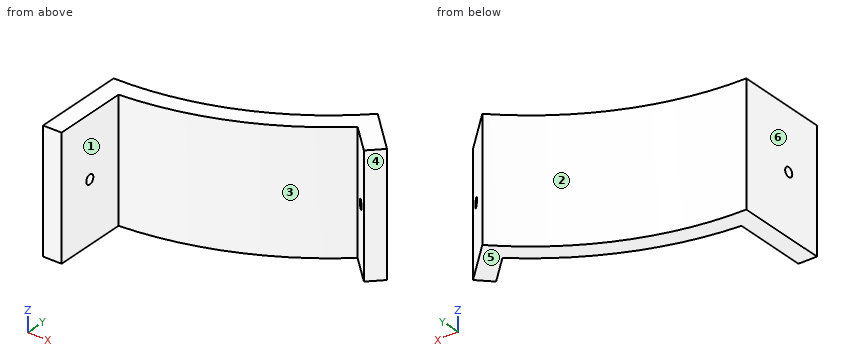
from build123d import *

# Parameters (mm, degrees)
SALIENTE_EXTRUIR1_DEPTH = 65.25
CROQUIS5_R              = 2.5
CORTAR_EXTRUIR3_DEPTH   = 45
CROQUIS6_R              = 2.5
CORTAR_EXTRUIR4_DEPTH   = 12


with BuildPart() as part:
    # Croquis1 → Saliente-Extruir1 (new body)
    with BuildSketch(Plane.XY):
        with BuildLine():
            Line((129.342755363, -129.342755363), (108.187337522, -108.187337522))
            ThreePointArc((108.187337522, -108.187337522), (58.550565152, -141.353568474), (0, -153))
            Line((0, -153), (0, -163))
            Line((0, -163), (0, -203))
            Line((0, -203), (10, -203))
            Line((10, -203), (10, -162.692962355))
            ThreePointArc((10, -162.692962355), (62.377399476, -150.592363799), (107.970229121, -122.112364745))
            Line((107.970229121, -122.112364745), (122.271687551, -136.413823175))
            Line((122.271687551, -136.413823175), (129.342755363, -129.342755363))
        make_face()
    extrude(amount=SALIENTE_EXTRUIR1_DEPTH)

    # Croquis5 → Cortar-Extruir3 (cut)
    with BuildSketch(Plane(origin=(10, 0, 0), x_dir=(0, 0, -1), z_dir=(1, 0, 0))):
        with Locations((-32.625, -183)):
            Circle(CROQUIS5_R)
    extrude(amount=-CORTAR_EXTRUIR3_DEPTH, mode=Mode.SUBTRACT)

    # Croquis6 → Cortar-Extruir4 (cut)
    with BuildSketch(Plane(origin=(0, 0, 0), x_dir=(0, 0, -1), z_dir=(0.707106781, 0.707106781, 0))):
        with Locations((-32.62, -172.768278829)):
            Circle(CROQUIS6_R)
    extrude(amount=-CORTAR_EXTRUIR4_DEPTH, mode=Mode.SUBTRACT)


solid = part.part
Source: CAD feature listing. Evaluate the final solid. Frame: model axes, mm. Face numbers are marked on the shaded views. A direction names the side the tool comes from. Coordinates: 2 decimals unless noted, no trailing zeros. Order: outer loops, then holes, each group sorted by start corner. A loop starts at its lowest first (then second) coordinate and runs counter-clockwise, first axis right, second up.
Item 1: Cut plane C-C (x = 87). Return loops of the section in (y, z).
Output values:
outline: (-137.84, 0) - (-125.86, 0) - (-125.86, 65.25) - (-137.84, 65.25) - close
Item 2: Material intervals for line 1 (Z direction, x = 8.25, y = -183) (3 decimals); line 2 (X direction, y = -173.5, z = 38); line 3 (X direction, y = -126, z = 48.5), sorted ascending.
Output values:
line 1: z = 0 to 30.125, 35.125 to 65.25
line 2: x = 0 to 10
line 3: x = 86.79 to 103.41, 111.86 to 126
Item 3: Cut plane B-B (z = 44.5). Return loops of the section in (x, y), plus the area to 3 significant figures.
Output values:
outline: (0, -203) - (10, -203) - (10, -162.69) arc R163 ccw to (107.97, -122.11) - (122.27, -136.41) - (129.34, -129.34) - (108.19, -108.19) arc R153 cw to (0, -153) - close
area: 1,840 mm2
Item 4: Cut plane A-A (y = -183). Return loops of the section in (x, z) (3 decimals).
Output values:
outline: (0, 0) - (10, 0) - (10, 30.125) - (0, 30.125) - close; (0, 35.125) - (10, 35.125) - (10, 65.25) - (0, 65.25) - close
Item 5: First-contact query: P1, Ø12, axis at x = 91.5, z = 14, coming from the -Y side; P2, Ø6, axis at y = -183, z = 32.625, coming from the +X side; P3, Ø8, axis at x = 76, z = 7.5, coming from the +Y side. Flat tips, straight axial feed; report the tip coordinate or a pass-through.
Output values:
P1: stops at y = -138.78
P2: stops at x = 10
P3: stops at y = -130.42
Item 6: Set-up query: the marked faces 1 and 2. Return all of +Z, -Z, +X, -X, +Y, -Y with unobstructed straight access to the full face (end or side cutting, diameter ignored); none if empty.
Output values:
face 1: +Z, -Z, +X, -Y
face 2: +Z, -Z, -X, +Y
Item 7: Pull-direction query (X, two-part tool) for the marked faces 3, 4, 5 and 6; classes: pulls with the +X half, pulls with the -X half, needs draft (parallel to the pull), parting line crosses it, or undercut.
Output values:
face 3: undercut
face 4: pulls with the +X half
face 5: needs draft
face 6: pulls with the -X half
Item 8: Cut plane D-D (y = -148). Return loops of the section in (x, z).
Output values:
outline: (38.79, 0) - (68.3, 0) - (68.3, 65.25) - (38.79, 65.25) - close
